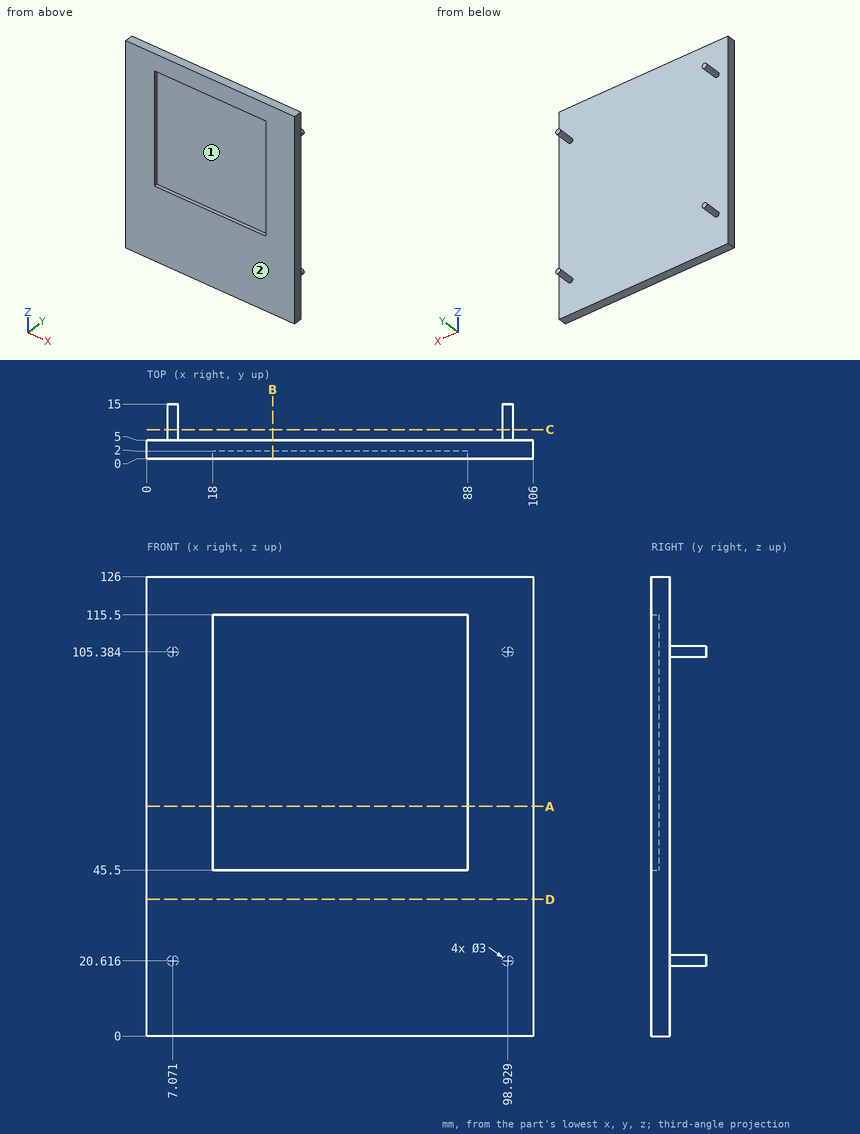
Drawing for the job (mm, zero at the part's lowest x, y, z). Round coordinates to 2 decimals unless told otherwise and drop trailing zeros. Loops run counter-clockwise (first coordinate to the right, second up) from the corner with the lowest first, then second, coordinate; pieces in that order, holes last. Notation, with made-up numbers: (17.25, 41.5) -> (65.25, 41.5) arc R19 cw to (65.25, 55.5) -> close; hole circle Ø3 at (78, 11.5). An arc over 180 degrees is marked (long way). Answer as CSV lines item,"result". Start each with the question number.
1) Slice it at A-A (z = 63). List the corners of the cut face in (x, y).
2) Slice it at D-D (z = 37.5). List the corners of the cut face in (x, y).
3) Slice it at C-C (y = 8). List the corners of the cut face in (x, z), plus the area to 3 significant figures.
4) Mould opens along X. For the marked faces 1 and 2 say: +X half, -X half, draft (parallel to the pull), parting line (faces both ways), or undercut.
5) Pin check, flat tips, straight feed: P1, Ø3, axis at x = 43, z = 23, coming from the +Y side; P2, Ø1.5, axis at x = 64, z = 49, coming from the -Y side; P3, Ø0.6, axis at y = 1, z = 86, coming from the -X side; P4, Ø6, axis at y = 10.5, z = 103, coming from the +X side. Stop position of each tip, or through.
6) Slice it at B-B (x = 34.5). List the corners of the cut face in (y, z), plus the area to 3 significant figures.
7) Probe line 1 along Y through (x, z) = (33, 82.5); line 2 along Y through (x, z) = (5, 13.5); line 3 along Z through (x, y) = (98.5, 12.25). List the from-to ranges inside material, lowest first.
Filled in:
1,outline,"(0, 0) -> (18, 0) -> (18, 2) -> (88, 2) -> (88, 0) -> (106, 0) -> (106, 5) -> (0, 5) -> close"
2,outline,"(0, 0) -> (106, 0) -> (106, 5) -> (0, 5) -> close"
3,outline,"circle Ø3 at (7.07, 20.62); circle Ø3 at (7.07, 105.38); circle Ø3 at (98.93, 20.62); circle Ø3 at (98.93, 105.38)"
3,area,"28.3 mm2"
4,face 1,"undercut"
4,face 2,"draft"
5,P1,"stops at y = 5"
5,P2,"stops at y = 2"
5,P3,"stops at x = 0"
5,P4,"stops at x = 100.43"
6,outline,"(0, 0) -> (5, 0) -> (5, 126) -> (0, 126) -> (0, 115.5) -> (2, 115.5) -> (2, 45.5) -> (0, 45.5) -> close"
6,area,"490 mm2"
7,line 1,"y = 2 to 5"
7,line 2,"y = 0 to 5"
7,line 3,"z = 19.18 to 22.05, 103.95 to 106.82"
